The drawing under review shows one solid part. Ordinate dimensions are in mm from its lowest x, y, z. A direction names the side the tool comes from. Coordinates: 2 decimals unless noted, no trailing zeros. Order: outer loops, then holes, each group sorted by start corner. A loop starts at its lowest first (then second) coordinate and runs counter-clockwise, first axis right, second up. Notation, with made-up numbers: M 41.5,42 L 50.5,42 A23 cw 50.5,59 Z; hole C -9.75,-14.75 d6. An arc over 180 degrees is marked long. Answer as a JSON object with one key per item and string values.
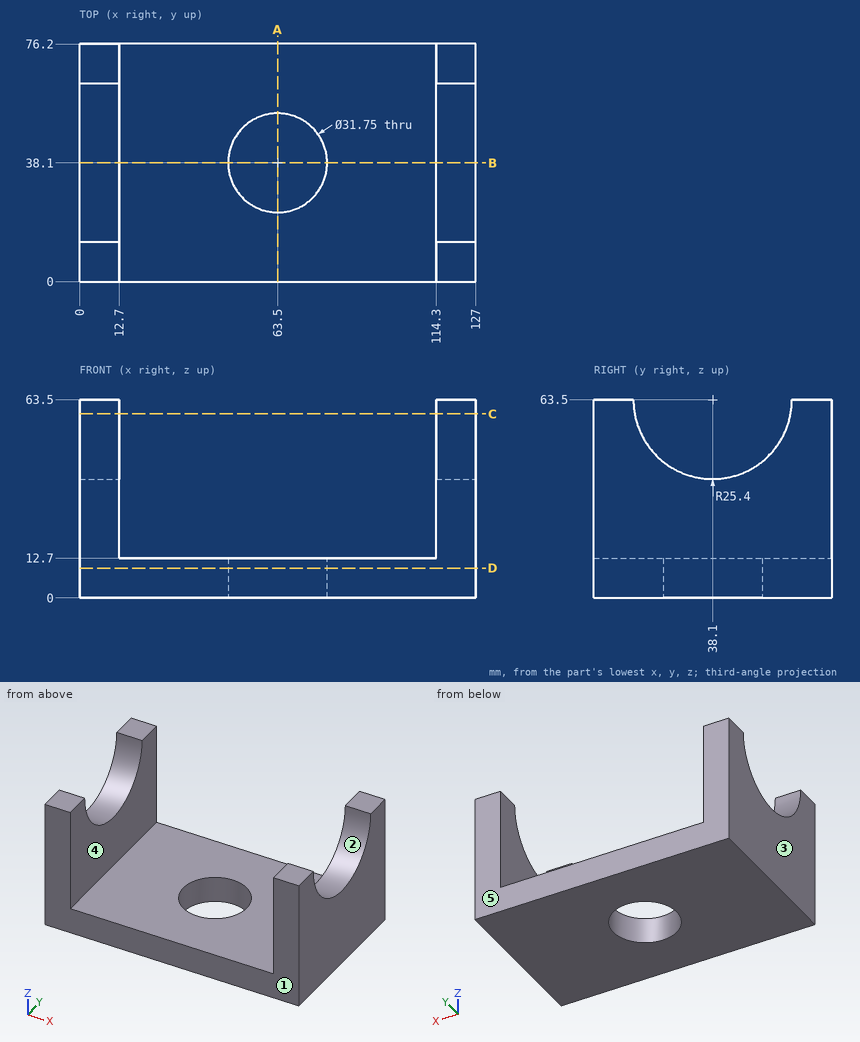
1) Tool access review of the marked faces 4 and 5: name each direction out of +Z, -Z, +X, -X, +Y, -Y from which nothing blocks a thin tool from reaching the whole face with its end or side.
Taken from the geometry:
{"face 4": "+Z, +Y, -Y", "face 5": "+Z, -Z, +X, -X, +Y"}
2) Insertion check: pin 1 Ø10 at (x, y) = (70, 14) entering from -Z; pin 2 Ø6 at (x, y) = (77, 9) entering from +Z. Each pin has a flat end and moves straight along its axis. Give the tip position at first contact, or say it passes through.
Taken from the geometry:
{"pin 1": "stops at z = 0", "pin 2": "stops at z = 12.7"}
3) Add section D-D (z = 9.5). State the section outline as (x, y) points (3 decimals).
Taken from the geometry:
{"outline": "M 0,0 L 127,0 L 127,76.2 L 0,76.2 Z; hole C 63.5,38.1 d31.75"}
4) To check wall thickness, follow L1, parallel to X at y = 70, z = 26; L2, parallel to Y at x = 63.5, z = 5.5 (3 decimals); L3, parallel to X at y = 38, z = 8. State the ranges of each line that lie inside material, in increasing order.
Taken from the geometry:
{"L1": "x = 0 to 12.7, 114.3 to 127", "L2": "y = 0 to 22.225, 53.975 to 76.2", "L3": "x = 0 to 47.63, 79.37 to 127"}
5) Add section C-C (z = 59). State the section outline as (x, y) points, and give its area (3 significant figures).
Taken from the geometry:
{"outline": "M 0,0 L 12.7,0 L 12.7,13.1 L 0,13.1 Z; M 0,63.1 L 12.7,63.1 L 12.7,76.2 L 0,76.2 Z; M 114.3,0 L 127,0 L 127,13.1 L 114.3,13.1 Z; M 114.3,63.1 L 127,63.1 L 127,76.2 L 114.3,76.2 Z", "area": "666 mm2"}
6) Add section B-B (y = 38.1). State the section outline as (x, z) points (3 decimals), and give its area (3 significant figures).
Taken from the geometry:
{"outline": "M 0,0 L 47.625,0 L 47.625,12.7 L 12.7,12.7 L 12.7,38.1 L 0,38.1 Z; M 79.375,0 L 127,0 L 127,38.1 L 114.3,38.1 L 114.3,12.7 L 79.375,12.7 Z", "area": "1,850 mm2"}
7) Mouldability with a two-part tool opening along Y and no side actions: class the marked faces 1, 2 and 3 as released by +Y, released by -Y, zero draft, split by the parting line, or undercut.
Taken from the geometry:
{"face 1": "released by -Y", "face 2": "undercut", "face 3": "zero draft"}
8) Add section A-A (x = 63.5). State the section outline as (y, z) points (3 decimals), and give its area (3 significant figures).
Taken from the geometry:
{"outline": "M 0,0 L 22.225,0 L 22.225,12.7 L 0,12.7 Z; M 53.975,0 L 76.2,0 L 76.2,12.7 L 53.975,12.7 Z", "area": "565 mm2"}
